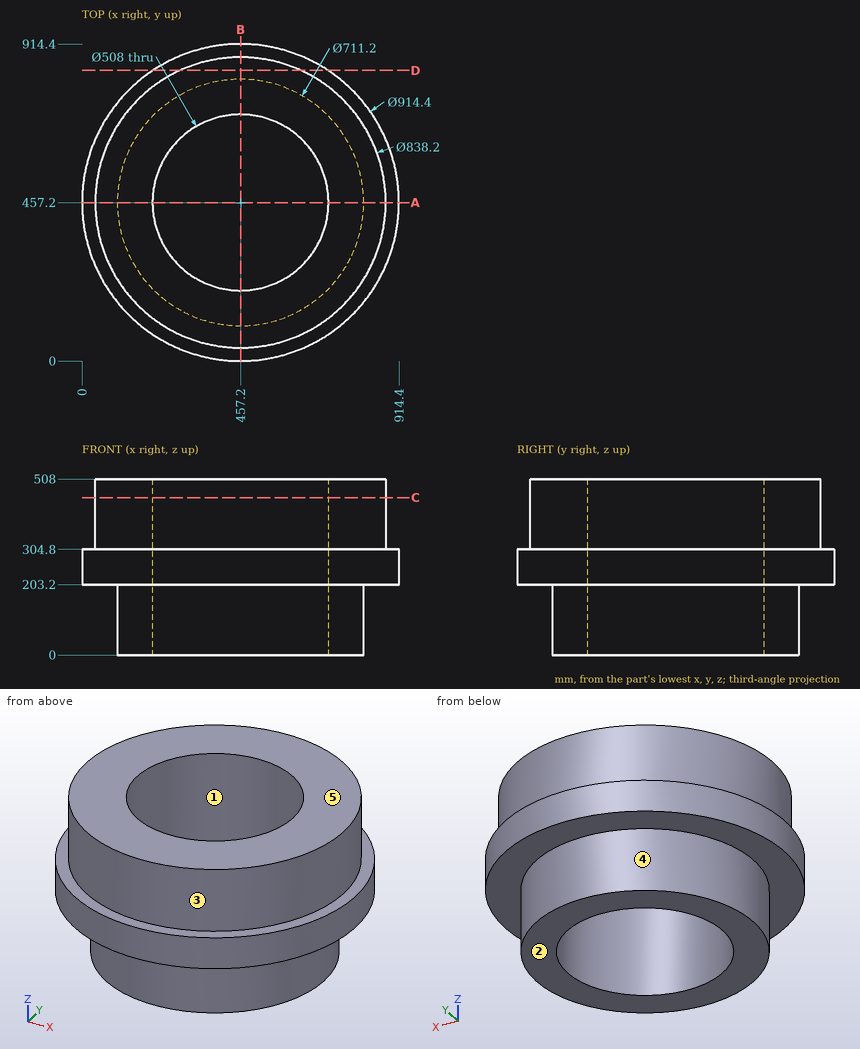
Part print with two shaded views. Sizes in mm from the minimum x, y, z corner. A direction names the side the tool comes from. Round coordinates to 2 decimals unless told otherwise and drop trailing zeros. Loops run counter-clockwise (first coordinate to the right, second up) from the corner with the lowest first, then second, coordinate; pieces in that order, holes last. Notation, with made-up numbers: (40, -24) - (86, -24) arc R20 ccw to (86, -7) - close; hole circle Ø10 at (20, 75.25). An arc over 180 degrees is marked (long way). Put each result on its own line as item: value.
1. Pin check, flat tips, straight feed: P1, Ø2, axis at x = 323.5, z = 95.5, coming from the +Y side; P2, Ø5, axis at y = 647, z = 180, coming from the -X side; P3, Ø4, axis at y = 557.5, z = 284.5, coming from the +X side. Stop position of each tip, or through.
Geometry check:
P1: y = 787.11
P2: x = 154.93
P3: x = 903.71
2. Two-plate mould, pull along Y, no slides. Class the marked faces 1, 2 and 3: released by +Y, released by -Y, zero draft, split by the parting line, or undercut.
Geometry check:
face 1: undercut
face 2: zero draft
face 3: split by the parting line
3. Slice it at A-A on y = 457.2. List the corners of the cut face in (x, z).
Geometry check:
outline: (0, 203.2) - (101.6, 203.2) - (101.6, 0) - (203.2, 0) - (203.2, 508) - (38.1, 508) - (38.1, 304.8) - (0, 304.8) - close; (711.2, 0) - (812.8, 0) - (812.8, 203.2) - (914.4, 203.2) - (914.4, 304.8) - (876.3, 304.8) - (876.3, 508) - (711.2, 508) - close
4. Wall check: line 1 (Y direction, x = 457.2, z = 210); line 2 (Y direction, x = 457.2, z = 182.5); line 3 (Z direction, x = 549, y = 801). Give the ranges that are in metal, low to high.
Geometry check:
line 1: 0 to 203.2, 711.2 to 914.4
line 2: 101.6 to 203.2, 711.2 to 812.8
line 3: 203.2 to 508
5. Slice it at D-D on y = 838. List the corners of the cut face in (x, z).
Geometry check:
outline: (204.17, 203.2) - (710.23, 203.2) - (710.23, 304.8) - (632.23, 304.8) - (632.23, 508) - (282.17, 508) - (282.17, 304.8) - (204.17, 304.8) - close
6. Slice it at C-C on z = 454.5. List the corners of the cut face in (x, y).
Geometry check:
outline: circle Ø838.2 at (457.2, 457.2); hole circle Ø508 at (457.2, 457.2)
7. 3-axis set-ups, long thin cutter, end or side, ignore diameter. For the marked faces 4 and 5: which of +Z, -Z, +X, -X, +Y, -Y reach the whole face in a straight line?
Geometry check:
face 4: -Z
face 5: +Z, +X, -X, +Y, -Y
